Autodesk Inventor part; units mm, degrees
ref_plane "YZ Plane" through (0, 0, 0) normal (1, 0, 0) x (0, 1, 0)
ref_plane "XZ Plane" through (0, 0, 0) normal (0, 1, 0) x (-1, 0, 0)
ref_plane "XY Plane" through (0, 0, 0) normal (0, 0, 1) x (1, 0, 0)
sketch "Sketch1" plane through (0, 0, 0) normal (0, 0, 1) x (1, 0, 0)
  circle A0 centre (0, 0) radius 50.8
extrude "Extrusion1" add sketch "Sketch1" along normal blind 38.1
sketch "Sketch2" plane through (0, 0, 38.1) normal (0, 0, 1) x (1, 0, 0)
  circle A0 centre (0, 0) radius 31.75 construction
  circle A1 centre (0, 0) radius 31.75 construction
  circle A2 centre (0, 0) radius 31.75 construction
  circle A3 centre (0, 0) radius 31.75 construction
  circle A4 centre (0, 0) radius 31.75 construction
  point P0 (0, 31.75)
  point P1 (-30.196, 9.8113)
  point P2 (-18.6622, -25.6863)
  point P3 (18.6622, -25.6863)
  point P4 (30.196, 9.8113)
  dimension "d8" = 63.5
  dimension "d11" = 360
hole "Hole1" at (0, 31.75, 38.1) direction (0, 0, -1) diameter 6.35 depth 38.1 tip angle 118
hole "Hole2" at (30.196, 9.8113, 38.1) direction (0, 0, -1) diameter 6.985 depth 38.1 tip angle 118 counterbore diameter 19.05 counterbore depth 6.35
hole "Hole3" at (18.6622, -25.6863, 38.1) direction (0, 0, -1) diameter 9.0678 end through all countersink diameter 19.05 countersink angle 82
hole "Hole4" at (-18.6622, -25.6863, 38.1) direction (0, 0, -1) diameter 4.9784 end through all
hole "Hole5" at (-30.196, 9.8113, 38.1) direction (0, 0, -1) diameter 13.4874 end through all
properties part number "Hole Practice"
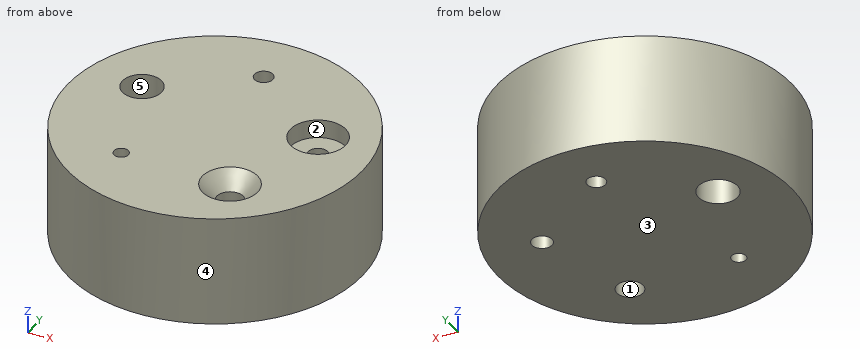
Source: CAD feature listing. Evaluate the final solid. Frame: model axes, mm. Face numbers are marked on the shaded views. A direction names the side the tool comes from. Coordinates: 2 decimals unless noted, no trailing zeros. Order: outer loops, then holes, each group sorted by start corner. A loop starts at its lowest first (then second) coordinate and runs counter-clockwise, first axis right, second up. Notation, with made-up numbers: (-36, 85.25) - (-29, 85.25) arc R18 ccw to (-29, 99.25) - close; hole circle Ø9 at (-24.5, -23.75). An arc over 180 degrees is marked (long way). One line per item, written item: value.
1) Cut plane D-D on z = 13. State how many separate pieces and enclosed holes the cut face has, plus the area to 3 significant figures.
Computed values:
separate pieces: 1
enclosed holes: 5
area: 7,810 mm^2
2) Cut plane C-C on x = 38. Output: boundary loops of the cut face in (y, z), plus the area to 3 significant figures.
Computed values:
outline: (-33.71, 0) - (33.71, 0) - (33.71, 38.1) - (15.27, 38.1) - (15.27, 31.75) - (4.35, 31.75) - (4.35, 38.1) - (-33.71, 38.1) - close
area: 2,500 mm^2
3) Ray query, line 1 (Y direction, x = 0, z = 21) (3 decimals); line 2 (X direction, y = -27, z = 28.5); line 3 (X direction, y = 30, z = 34). Return the intervals inside material, ascending. Write a range as [from, to].
Computed values:
line 1: y = [-50.8, 28.575], [34.925, 50.8]
line 2: x = [-43.03, -20.78], [-16.55, 14.32], [23, 43.03]
line 3: x = [-41, -2.65], [2.65, 41]
4) Contact query for flat-ended pins moving along their axis: pin 1 (4 mm diameter, centred on y = 6, z = 13, fed in from +X); pin 2 (1.5 mm diameter, centred on y = -33.5, z = 8, fed in from -X); pin 3 (12 mm diameter, centred on x = -30.2, y = 9.81, fed in from +Z); pin 4 (4 mm diameter, centred on x = -36.5, z = 16, fed in from +Y). Output: stop coordinate, or through.
Computed values:
pin 1: stops at x = 50.64
pin 2: stops at x = -38.83
pin 3: passes through
pin 4: stops at y = 37.29
5) Reachability of the marked faces 1 and 2 from +Z, -Z, +X, -X, +Y, -Y: full face, straight path, thin tool, end or side. Return the list, or none.
Computed values:
face 1: +Z, -Z
face 2: +Z
6) Mould query, pull axis X, two halves, no side actions, for the marked faces 3, 4 and 5. Classes: released by +X, released by -X, zero draft, split by the parting line, or undercut.
Computed values:
face 3: zero draft
face 4: split by the parting line
face 5: undercut
7) Cut plane B-B on y = 31.75. Output: boundary loops of the cut face in (x, z) (3 decimals).
Computed values:
outline: (-39.656, 0) - (-3.175, 0) - (-3.175, 38.1) - (-39.656, 38.1) - close; (3.175, 0) - (39.656, 0) - (39.656, 38.1) - (3.175, 38.1) - close
8) Cut plane A-A on x = 0. Output: boundary loops of the cut face in (y, z) (3 decimals).
Computed values:
outline: (-50.8, 0) - (28.575, 0) - (28.575, 38.1) - (-50.8, 38.1) - close; (34.925, 0) - (50.8, 0) - (50.8, 38.1) - (34.925, 38.1) - close
